Could you check a few things on this model? Use its own coordinates, in mm. Face numbers are marked on the shaded views. A direction names the side the tool comes from. Give positions to 0.01 mm unless a question says otherwise; leave off trailing zeros. Loops run counter-clockwise (first coordinate to the right, second up) from the corner with the lowest first, then second, coordinate; pieces in that order, holes last. Notation, with made-up numbers: (61.25, 13.25) -> (67.25, 13.25) arc R20 cw to (67.25, 25.25) -> close; hole circle Ø5 at (23, 27). An arc over 180 degrees is marked (long way). Write each question's results on one line, items separated by ' | '. Start each with the question number.
Q1. If we section it at A-A, the plane x = 59: List the corners of the cut face in (y, z) for me.
Q2. If we section it at C-C, the plane y = 3: List the corners of the cut face in (x, z) for me.
Q3. If we section it at D-D, the plane x = 24: List the corners of the cut face in (y, z) for me, plus the area to 3 significant figures.
Q4. If I drill on line 1 along Z through (x, y) = (52, -4.25); line 2 along Z through (x, y) = (32, 3.75); line 3 along X through (y, z) = (-13.75, -21), over which ranges is the centre line in solid material (lowest first)?
Q5. Which directions (+Z, -Z, +X, -X, +Y, -Y) give clear straight access to the entire face, cutting with the end or side of a thin tool? Please do the marked faces 5, 6, 7 and 8.
Q6. If we section it at B-B, the plane z = -20: List the corners of the cut face in (x, y) for me (3 decimals).
Q7. Will these pins go through, and if not, where does the flat tip stop? P1, Ø4, axis at x = 26.5, y = 6.5, coming from the +Z side; P2, Ø3, axis at y = -10, z = -9, coming from the +X side; P3, Ø1.5, axis at x = 53.5, y = -6, coming from the -Z side.
Q8. We'd pull the mould along X, two halves only. Please class the marked faces 1, 2, 3 and 4: released by +X, released by -X, zero draft, split by the parting line, or undercut.
from build123d import *

# Parameters (mm, degrees)
SKETCH1_W           = 80.01
SKETCH1_H           = 36.068
SKETCH1_R           = 1.5875
PCB_DEPTH           = 1.5494
SKETCH2_W           = 71.628
SKETCH2_H           = 26.924
BOSS_EXTRUDE2_DEPTH = 7.62
SKETCH3_W           = 64.262
SKETCH3_H           = 13.843
SCREEN_DEPTH        = 1.016
SKETCH4_W           = 48.133
SKETCH4_H           = 28.6512
CIRCUITS_DEPTH      = 13.462
SKETCH5_W           = 0.635
SKETCH5_H           = 0.635
PINS_DEPTH          = 2.54


with BuildPart() as part:
    # Sketch1 → PCB (new body)
    with BuildSketch(Plane(origin=(0, 0, 0), x_dir=(1, 0, 0), z_dir=(0, 1, 0))):
        with Locations((40.005, 18.034)):
            Rectangle(SKETCH1_W, SKETCH1_H)
        with Locations((2.3495, 2.3495)):
            Circle(SKETCH1_R, mode=Mode.SUBTRACT)
        with Locations((77.6605, 2.3495)):
            Circle(SKETCH1_R, mode=Mode.SUBTRACT)
        with Locations((77.6605, 33.7185)):
            Circle(SKETCH1_R, mode=Mode.SUBTRACT)
        with Locations((2.3495, 33.7185)):
            Circle(SKETCH1_R, mode=Mode.SUBTRACT)
    extrude(amount=PCB_DEPTH)

    # Sketch2 → Boss-Extrude2 (add)
    with BuildSketch(Plane(origin=(0, 1.5494, 0), x_dir=(1, 0, 0), z_dir=(0, 1, 0))):
        with Locations((40.386, 17.526)):
            Rectangle(SKETCH2_W, SKETCH2_H)
    extrude(amount=BOSS_EXTRUDE2_DEPTH)

    # Sketch3 → Screen (cut)
    with BuildSketch(Plane(origin=(0, 9.1694, 0), x_dir=(1, 0, 0), z_dir=(0, 1, 0))):
        with Locations((40.386, 17.526)):
            Rectangle(SKETCH3_W, SKETCH3_H)
    extrude(amount=-SCREEN_DEPTH, mode=Mode.SUBTRACT)

    # Sketch4 → Circuits (add)
    with BuildSketch(Plane.XZ):
        with Locations((30.4165, -21.2344)):
            Rectangle(SKETCH4_W, SKETCH4_H)
    extrude(amount=CIRCUITS_DEPTH)

    # Sketch5 → Pins (add)
    with BuildSketch(Plane.XZ.offset(13.462)):
        with Locations((8.382, -18.6436)):
            Rectangle(SKETCH5_W, SKETCH5_H)
        with Locations((8.382, -21.1836)):
            Rectangle(SKETCH5_W, SKETCH5_H)
        with Locations((8.382, -23.7236)):
            Rectangle(SKETCH5_W, SKETCH5_H)
    extrude(amount=PINS_DEPTH)


solid = part.part
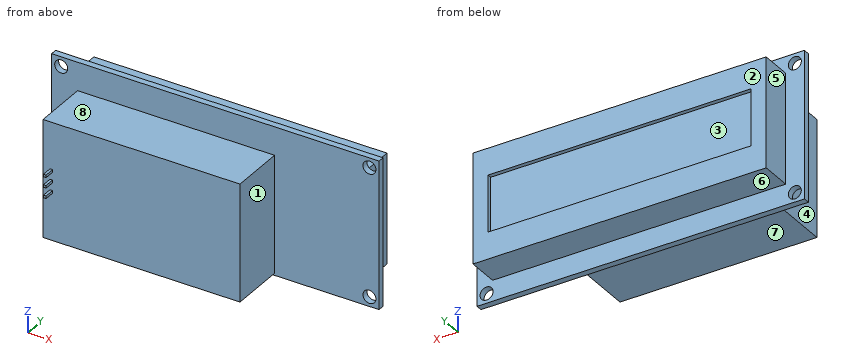
Final values:
1) outline: (0, -36.07) -> (1.55, -36.07) -> (1.55, -30.99) -> (9.17, -30.99) -> (9.17, -24.45) -> (8.15, -24.45) -> (8.15, -10.6) -> (9.17, -10.6) -> (9.17, -4.06) -> (1.55, -4.06) -> (1.55, 0) -> (0, 0) -> close
2) outline: (4.57, -30.99) -> (76.2, -30.99) -> (76.2, -4.06) -> (4.57, -4.06) -> close
3) outline: (-13.46, -35.56) -> (0, -35.56) -> (0, -36.07) -> (1.55, -36.07) -> (1.55, -30.99) -> (9.17, -30.99) -> (9.17, -24.45) -> (8.15, -24.45) -> (8.15, -10.6) -> (9.17, -10.6) -> (9.17, -4.06) -> (1.55, -4.06) -> (1.55, 0) -> (0, 0) -> (0, -6.91) -> (-13.46, -6.91) -> close | area: 633 mm²
4) line 1: z = -35.56 to -6.91 | line 2: z = -30.99 to -4.06 | line 3: x = 8.06 to 8.7
5) face 5: +Z, -Z, -X, +Y | face 6: -Z, +X, -X, +Y | face 7: -Z, +X, -X, -Y | face 8: +Z, +X, -X, -Y
6) outline: (0, 0) -> (6.35, 0) -> (6.35, -13.462) -> (54.483, -13.462) -> (54.483, 0) -> (80.01, 0) -> (80.01, 1.549) -> (76.2, 1.549) -> (76.2, 9.169) -> (72.517, 9.169) -> (72.517, 8.153) -> (8.255, 8.153) -> (8.255, 9.169) -> (4.572, 9.169) -> (4.572, 1.549) -> (0, 1.549) -> close
7) P1: stops at z = -4.06 | P2: stops at x = 54.48 | P3: stops at z = -35.56
8) face 1: released by +X | face 2: zero draft | face 3: undercut | face 4: released by -X
